Input: part model. Units: mm. Frame: model coordinates. A direction names the side the tool comes from. Coordinates: 2 decimals unless noted, no trailing zeros. Loops run counter-clockwise (first coordinate to the right, second up) from the corner with the lowest first, then second, coordinate; pieces in that order, holes last.
Item 1: Contact query for flat-ended pins moving along their axis: P1, Ø15, axis at x = 481.5, z = 635.5, coming from the +Y side; P2, Ø7.5, axis at y = 821, z = 435.5, coming from the -X side; P3, Ø8, axis at x = 591, y = 546.5, coming from the +Z side; P4, Ø2, axis at x = 222, y = 686, coming from the -Z side. Output: stop coordinate, or through.
Item 2: Section D-D on x = 593.5. Return loops of the section in (y, z).
Item 3: Section A-A on x = 393.5. Return loops of the section in (y, z).
Item 4: Section B-B on z = 281. Return loops of the section in (x, y), and give its area (3 significant figures).
Item 5: Section C-C on y = 750. Return loops of the section in (x, z), and give its area (3 significant figures).
Item 6: Ray query, line 1 along Y through (x, z) = (-88, 676.5); line 2 along Z through (x, y) = (-74.5, 728.5); line 3 along Y through (x, z) = (190, 129). Return the intervals inside material, ascending.
Item 7: Reachability of faces 1 (the flat face through (771.692, 631, 330)), 2 (the flat face through (308, 635, 0)), 3 (the flat face through (302, 823, 438.796)), 4 (the flat face through (152.141, 823, 339)), 5 (the flat face through (302, 823, 235.596)) from +Z, -Z, +X, -X, +Y, -Y: full face, straight path, thin tool, end or side. Return the list, or none.
```python
from build123d import *

# Parameters (mm, degrees)
SKETCH2_W           = 914.4
SKETCH2_H           = 304.8
BOSS_EXTRUDE3_DEPTH = 609.6
SKETCH3_W           = 914.4
SKETCH3_H           = 244.302361722
BOSS_EXTRUDE4_DEPTH = 50.8
SKETCH4_W           = 914.4
SKETCH4_H           = 189.735334449
BOSS_EXTRUDE5_DEPTH = 50.8
SKETCH5_W           = 914.4
SKETCH5_H           = 141.869521053
BOSS_EXTRUDE6_DEPTH = 50.8
SKETCH6_W           = 914.4
SKETCH6_H           = 88.259810048
BOSS_EXTRUDE7_DEPTH = 50.8
SKETCH7_W           = 914.4
SKETCH7_H           = 44.129905024
BOSS_EXTRUDE8_DEPTH = 50.8
SKETCH8_W           = 304.8
SKETCH8_H           = 203.2
BOSS_EXTRUDE9_DEPTH = 76.2
SKETCH9_W           = 70
SKETCH9_H           = 30
CUT_EXTRUDE1_DEPTH  = 6.604


with BuildPart() as part:
    # Sketch2 → Boss-Extrude3 (new body)
    with BuildSketch(Plane.XY):
        with Locations((314.492107476, 633.364976232)):
            Rectangle(SKETCH2_W, SKETCH2_H)
    extrude(amount=BOSS_EXTRUDE3_DEPTH)

    # Sketch3 → Boss-Extrude4 (add)
    with BuildSketch(Plane.XY.offset(609.6)):
        with Locations((314.492107476, 603.116157093)):
            Rectangle(SKETCH3_W, SKETCH3_H)
    extrude(amount=BOSS_EXTRUDE4_DEPTH)

    # Sketch4 → Boss-Extrude5 (add)
    with BuildSketch(Plane.XY.offset(660.4)):
        with Locations((314.492107476, 575.832643457)):
            Rectangle(SKETCH4_W, SKETCH4_H)
    extrude(amount=BOSS_EXTRUDE5_DEPTH)

    # Sketch5 → Boss-Extrude6 (add)
    with BuildSketch(Plane.XY.offset(711.2)):
        with Locations((314.492107476, 551.899736759)):
            Rectangle(SKETCH5_W, SKETCH5_H)
    extrude(amount=BOSS_EXTRUDE6_DEPTH)

    # Sketch6 → Boss-Extrude7 (add)
    with BuildSketch(Plane.XY.offset(762)):
        with Locations((314.492107476, 525.094881256)):
            Rectangle(SKETCH6_W, SKETCH6_H)
    extrude(amount=BOSS_EXTRUDE7_DEPTH)

    # Sketch7 → Boss-Extrude8 (add)
    with BuildSketch(Plane.XY.offset(812.8)):
        with Locations((314.492107476, 503.029928744)):
            Rectangle(SKETCH7_W, SKETCH7_H)
    extrude(amount=BOSS_EXTRUDE8_DEPTH)

    # Sketch8 → Boss-Extrude9 (add)
    with BuildSketch(Plane(origin=(0, 785.764976232, 0), x_dir=(1, 0, 0), z_dir=(0, 1, 0))):
        with Locations((304.540679121, -337.195909304)):
            Rectangle(SKETCH8_W, SKETCH8_H)
    extrude(amount=BOSS_EXTRUDE9_DEPTH)

    # Sketch9 → Cut-Extrude1 (cut)
    with BuildSketch(Plane.XY.offset(438.795909304)):
        with Locations((379.707122213, 827.488030004)):
            Rectangle(SKETCH9_W, SKETCH9_H)
    extrude(amount=-CUT_EXTRUDE1_DEPTH, mode=Mode.SUBTRACT)


solid = part.part
```
Results found:
1. P1: stops at y = 725.27
1. P2: stops at x = 152.14
1. P3: stops at z = 812.8
1. P4: stops at z = 0
2. outline: (480.96, 0) - (785.76, 0) - (785.76, 609.6) - (725.27, 609.6) - (725.27, 660.4) - (670.7, 660.4) - (670.7, 711.2) - (622.83, 711.2) - (622.83, 762) - (569.22, 762) - (569.22, 812.8) - (525.09, 812.8) - (525.09, 863.6) - (480.96, 863.6) - close
3. outline: (480.96, 0) - (785.76, 0) - (785.76, 235.6) - (861.96, 235.6) - (861.96, 438.8) - (842.49, 438.8) - (842.49, 432.19) - (812.49, 432.19) - (812.49, 438.8) - (785.76, 438.8) - (785.76, 609.6) - (725.27, 609.6) - (725.27, 660.4) - (670.7, 660.4) - (670.7, 711.2) - (622.83, 711.2) - (622.83, 762) - (569.22, 762) - (569.22, 812.8) - (525.09, 812.8) - (525.09, 863.6) - (480.96, 863.6) - close
4. outline: (-142.71, 480.96) - (771.69, 480.96) - (771.69, 785.76) - (456.94, 785.76) - (456.94, 861.96) - (152.14, 861.96) - (152.14, 785.76) - (-142.71, 785.76) - close
4. area: 302,000 mm2
5. outline: (-142.71, 0) - (771.69, 0) - (771.69, 609.6) - (-142.71, 609.6) - close
5. area: 557,000 mm2
6. line 1: y = 480.96 to 670.7
6. line 2: z = 0 to 609.6
6. line 3: y = 480.96 to 785.76
7. face 1: +Z, -Z, +X, +Y, -Y
7. face 2: -Z, +X, -X, +Y, -Y
7. face 3: +Z, +X, -X, +Y
7. face 4: +Z, -Z, -X, +Y
7. face 5: -Z, +X, -X, +Y
